Autodesk Inventor part; units mm, degrees
ref_plane "YZ Plane" through (0, 0, 0) normal (1, 0, 0) x (0, 1, 0)
ref_plane "XZ Plane" through (0, 0, 0) normal (0, 1, 0) x (-1, 0, 0)
ref_plane "XY Plane" through (0, 0, 0) normal (0, 0, 1) x (1, 0, 0)
sketch "Sketch1" plane through (0, 0, 0) normal (1, 0, 0) x (0, 1, 0)
  arc A0 (-0.635, -11.743) -> (7.62, -8.9576) centre (0, 0) ccw
  arc A1 (-0.635, -7.5935) -> (6.0473, -4.6363) centre (0, 0) ccw
  circle A2 centre (7.62, -3.048) radius 2.2352
  line L0 (7.62, -5.2832) -> (7.62, -8.9576)
  line L1 (-0.635, -11.743) -> (-0.635, -7.5935)
  dimension "d0" = 11.7602
  dimension "d1" = 7.62
  dimension "d8" = 2.2352
  dimension "d9" = 7.62
  dimension "d10" = 3.048
  dimension "d11" = 0.635
extrude "Extrusion1" add sketch "Sketch1" along normal blind 5.7912
fillet "Fillet1" radius 1.27 1 edges at (2.8956, 6.0473, -4.6363)
fillet "Fillet2" radius 0.889 1 edges at (2.8956, 7.62, -5.2832)
fillet "Fillet3" radius 0.889 1 edges at (2.8956, 7.62, -8.9576)
ref_plane "Work Plane1" through (1.016, 0, 0) normal (-1, 0, 0) x (0, 0, 1)
sketch "Sketch2" plane through (1.016, 0, 0) normal (-1, 0, 0) x (0, 0, 1)
  arc A0 (-3.9958, 5.5957) -> (-5.4412, 5.3346) centre (-4.5343, 4.4455) ccw
  arc A1 (-5.4412, 5.3346) -> (-7.5935, -0.635) centre (0, 0) ccw
  line L0 (-7.5935, -0.635) -> (-11.743, -0.635)
  arc A2 (-9.2349, 7.2814) -> (-11.743, -0.635) centre (0, 0) ccw
  arc A3 (-8.5368, 7.62) -> (-9.2349, 7.2814) centre (-8.5368, 6.731) ccw
  line L1 (-8.5368, 7.62) -> (-6.043, 7.62)
  arc A4 (-6.043, 7.62) -> (-5.1908, 8.256) centre (-6.043, 8.509) ccw
  arc A5 (-3.9958, 5.5957) -> (-5.1908, 8.256) centre (-3.048, 7.62) ccw
  circle A6 centre (-10.414, -1.27) radius 1.397
  circle A7 centre (-0.635, 9.144) radius 1.397
  dimension "d18" = 1.397
  dimension "d19" = 1.27
  dimension "d20" = 10.414
  dimension "d21" = 1.397
  dimension "d22" = 0.635
  dimension "d23" = 9.144
extrude "Extrusion2" add sketch "Sketch2" against normal blind 2.032 contours A7 A5 | A5 A7 | A6 L0 | L0 A6
fillet "Fillet4" radius 1.27 1 edges at (2.8956, -0.635, -7.5935)
sketch "Sketch3" plane through (3.048, 0, 0) normal (1, 0, 0) x (0, 0, -1)
  arc A0 (1.9639, 9.5747) -> (0.8171, 7.7589) centre (0.635, 9.144) ccw
  line L0 (9.1697, -0.635) -> (11.6583, -0.635)
  arc A1 (9.1697, -0.635) -> (11.6583, -0.635) centre (10.414, -1.27) ccw
  point P0 (0, 0)
hole "Hole1" at (3.048, -1.27, -10.414) at (3.048, 9.144, -0.635) direction (-1, 0, 0) diameter 1.016 end through all
sketch "Sketch4" plane through (5.7912, 0, 0) normal (1, 0, 0) x (0, 0, -1)
  arc A0 (5.1908, 8.256) -> (3.9958, 5.5957) centre (3.048, 7.62) ccw
hole "Hole2" at (5.7912, 7.62, -3.048) direction (-1, 0, 0) diameter 2.032 end through all
properties part number "Brake Pad"
Could you check a few things on this model? Use its own coordinates, in mm. A direction names the side the tool comes from. Coordinates: 2 decimals unless noted, no trailing zeros. Order: outer loops, then holes, each group sorted by start corner. A loop starts at its lowest first (then second) coordinate and runs counter-clockwise, first axis right, second up.
Q1. Thinking about a two-plate mould opening in Z: for faces 6 (the cylindrical face through (2.018, 9.595, -0.869)), 7 (the cylindrical face through (2.936, 7.801, -5.505)), 8 (the flat face through (3, 7.62, -7)), which applies, released by +Z, released by -Z, zero draft, split by the parting line, or undercut?
Q2. Please list where these lines run through material, in increasing order: L1, parallel to Z at x = 1.5, y = -1.27; L2, parallel to Z at x = 2.7, y = 6.75; L3, parallel to X at y = -1.5, z = -9.25.
Q3. Suppose I cut it at D-D on y = 3.5. Please give me the cut outline in (x, z).
Q4. Will these pins go through, and if not, where does the flat tip stop? pin 1 (2.5 mm diameter, centred on x = 1.5, z = -7.5, fed in from +Y); pin 2 (1.6 mm diameter, centred on y = -1.5, z = -10.5, fed in from -X); pin 3 (2 mm diameter, centred on x = 1.5, z = -4.5, fed in from -Y).
Q5. Which directions (+Z, -Z, +X, -X, +Y, -Y) give clear straight access to the entire face, cutting with the end or side of a thin tool? Please do faces 1 (the flat face through (3.048, 9.5, 0)), 2 (the flat face through (1.016, -2, -10)), 3 (the flat face through (3.048, -2, -10)), 4 (the cylindrical face through (2.86, 8.52, -3.52)), 5 (the flat face through (1.016, 9.5, 0)).
Q6. Suppose I cut it at A-A on y = -1.27. Please give me the cut outline in (x, z), and give its area (3 significant figures).
Q7. Suppose I cut it at C-C on x = 1.9. Give the number of separate pieces and of enclosed holes in the cut face, and give its area (3 significant figures).
Q8. Suppose I cut it at B-B on z = -0.5. Please give me the cut outline in (x, y).
Answer:
1. face 6: undercut
1. face 7: released by -Z
1. face 8: zero draft
2. L1: z = -11.81 to -10.92, -9.91 to -9.02
2. L2: z = -9.63 to -3.57, -2.52 to -0.99
2. L3: x = 1.02 to 3.05
3. outline: (0, -11.23) - (5.79, -11.23) - (5.79, -6.77) - (0, -6.77) - close
4. pin 1: stops at y = 7.62
4. pin 2: stops at x = 1.02
4. pin 3: stops at y = 5.27
5. face 1: +Z, +X, +Y
5. face 2: +Z, -Z, -X, -Y
5. face 3: +Z, -Z, +X, -Y
5. face 4: +X, -X
5. face 5: +Z, -X, +Y
6. outline: (1.02, -11.81) - (3.05, -11.81) - (3.05, -10.92) - (1.02, -10.92) - close; (1.02, -9.91) - (3.05, -9.91) - (3.05, -9.02) - (1.02, -9.02) - close
6. area: 3.61 mm2
7. separate pieces: 1
7. enclosed holes: 3
7. area: 57.4 mm2
8. outline: (1.02, 7.75) - (3.05, 7.75) - (3.05, 8.65) - (1.02, 8.65) - close; (1.02, 9.63) - (3.05, 9.63) - (3.05, 10.53) - (1.02, 10.53) - close
